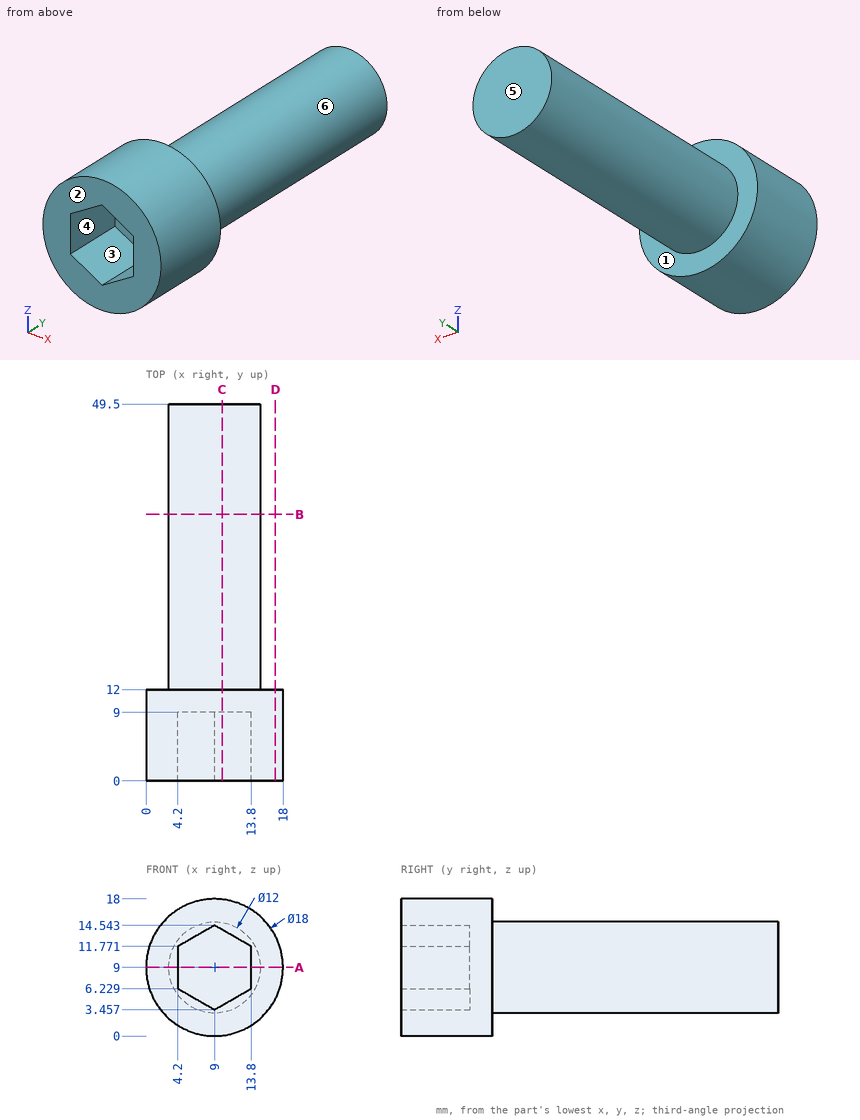
The drawing under review shows one solid part. Ordinate dimensions are in mm from its lowest x, y, z. A direction names the side the tool comes from. Coordinates: 2 decimals unless noted, no trailing zeros. Order: outer loops, then holes, each group sorted by start corner. A loop starts at its lowest first (then second) coordinate and runs counter-clockwise, first axis right, second up. Notation, with made-up numbers: (2.5, 3) -> (48.5, 3) arc R23 ccw to (48.5, 11) -> close; hole circle Ø9 at (49, -20). An arc over 180 degrees is marked (long way). One line per item, written item: value.
1) We need section B-B, the plane y = 35. Give the boundary of the cut face in (x, z).
Output values:
outline: circle Ø12 at (9, 9)
2) To check wall thickness, follow probe 1 along Y at (x, z) = (7.25, 13); probe 2 along Y at (x, z) = (16.25, 8.75); probe 3 along Z at (x, y) = (6.5, 3) (1 decimal). State the ranges of each line that lie inside material, in increasing order. Write a range as [from, to].
Output values:
probe 1: y = [9, 49.5]
probe 2: y = [0, 12]
probe 3: z = [0.4, 4.9], [13.1, 17.6]
3) Clearance check with flat-ended pins moving along their axes: P1, Ø10, axis at y = 33, z = 2, coming from the +X side; P2, Ø6, axis at y = 11.5, z = 12, coming from the -X side; P3, Ø4, axis at y = 42.5, z = 2, coming from the +X side (1 decimal); P4, Ø2, axis at x = 8, z = 7.5, coming from the -Y side. State where each tip first meets the part, or that it passes through.
Output values:
P1: stops at x = 14.66
P2: stops at x = 0
P3: stops at x = 12.3
P4: stops at y = 9
4) Draft analysis for pull direction Z (two halves, no side actions). For the marked faces 4, 5 and 6, state which applies: +Z half, -Z half, draft (parallel to the pull), parting line (faces both ways), or undercut.
Output values:
face 4: undercut
face 5: draft
face 6: parting line
5) We need section D-D, the plane x = 17. Give the boundary of the cut face in (y, z).
Output values:
outline: (0, 4.88) -> (12, 4.88) -> (12, 13.12) -> (0, 13.12) -> close
6) Machinability: for the marked faces 1, 2 and 3, which of the approach directions +Z, -Z, +X, -X, +Y, -Y give a long, thin tool a straight path to every point of the face, cutting with its end or side? Answer none if there is none.
Output values:
face 1: +Y
face 2: +Z, -Z, +X, -X, -Y
face 3: -Y
7) We need section C-C, the plane x = 10. Give the boundary of the cut face in (y, z) (1 decimal).
Output values:
outline: (0, 0.1) -> (12, 0.1) -> (12, 3.1) -> (49.5, 3.1) -> (49.5, 14.9) -> (12, 14.9) -> (12, 17.9) -> (0, 17.9) -> (0, 14) -> (9, 14) -> (9, 4) -> (0, 4) -> close
8) We need section A-A, the plane z = 9. Give the boundary of the cut face in (x, y).
Output values:
outline: (0, 0) -> (4.2, 0) -> (4.2, 9) -> (13.8, 9) -> (13.8, 0) -> (18, 0) -> (18, 12) -> (15, 12) -> (15, 49.5) -> (3, 49.5) -> (3, 12) -> (0, 12) -> close
